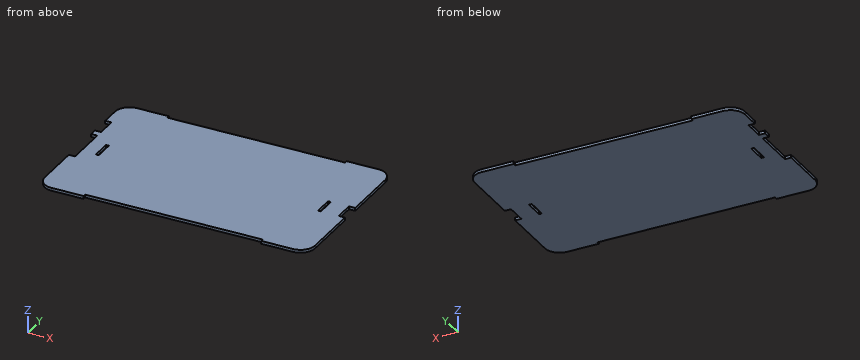
```python
from build123d import *

# Parameters (mm, degrees)
SALIENTE_EXTRUIR2_DEPTH = 3
CROQUIS2_W              = 6.5
CROQUIS2_H              = 20.5
CROQUIS2_H_2            = 44.2
CROQUIS2_W_2            = 3
CROQUIS2_H_3            = 20
CORTAR_EXTRUIR1_DEPTH   = 3


with BuildPart() as part:
    # Croquis1 → Saliente-Extruir2 (new body)
    with BuildSketch(Plane.XY):
        with BuildLine():
            Line((-207.344846765, 3), (-174.444846765, 3))
            Line((-174.444846765, 3), (-174.444846765, 0))
            Line((-174.444846765, 0), (9.755153235, 0))
            Line((9.755153235, 0), (9.755153235, 3))
            Line((9.755153235, 3), (42.655153235, 3))
            ThreePointArc((42.655153235, 3), (53.261754953, -1.393398282), (57.655153235, -12))
            Line((57.655153235, -12), (57.655153235, -152))
            ThreePointArc((57.655153235, -152), (53.261754953, -162.606601718), (42.655153235, -167))
            Line((42.655153235, -167), (9.755153235, -167))
            Line((9.755153235, -167), (9.755153235, -164))
            Line((9.755153235, -164), (-174.444846765, -164))
            Line((-174.444846765, -164), (-174.444846765, -167))
            Line((-174.444846765, -167), (-207.344846765, -167))
            ThreePointArc((-207.344846765, -167), (-217.951448483, -162.606601718), (-222.344846765, -152))
            Line((-222.344846765, -152), (-222.344846765, -12))
            ThreePointArc((-222.344846765, -12), (-217.951448483, -1.393398282), (-207.344846765, 3))
        make_face()
    extrude(amount=SALIENTE_EXTRUIR2_DEPTH)

    # Croquis2 → Cortar-Extruir1 (cut)
    with BuildSketch(Plane.XY.offset(3)):
        with Locations((-219.094846765, -42)):
            Rectangle(CROQUIS2_W, CROQUIS2_H)
        with Locations((-219.094846765, -82)):
            Rectangle(CROQUIS2_W, CROQUIS2_H_2)
        with Locations((54.405153235, -82)):
            Rectangle(CROQUIS2_W, CROQUIS2_H)
        with Locations((-199.094846765, -82)):
            Rectangle(CROQUIS2_W_2, CROQUIS2_H_3)
        with Locations((31.155153235, -82)):
            Rectangle(CROQUIS2_W_2, CROQUIS2_H_3)
    extrude(amount=-CORTAR_EXTRUIR1_DEPTH, mode=Mode.SUBTRACT)


solid = part.part
```
Part model, mm, in its own coordinate system. Round coordinates to 2 decimals unless told otherwise and drop trailing zeros. Write each loop counter-clockwise with the first axis right and the second up, starting at its lowest first coordinate (ties: lowest second). Pieces come first, ordered by that corner, then holes. Notation, with made-up numbers: (-12.75, 80) -> (19.25, 80) arc R21 ccw to (19.25, 108) -> close; hole circle Ø1 at (34, 40.5). An arc over 180 degrees is marked (long way). Return JSON: item names as keys, results as strings. Group by question number.
Q1. Pin check, flat tips, straight feed: pin 1 (1 mm diameter, centred on y = -34, z = 1, fed in from -X); pin 2 (12 mm diameter, centred on x = -136.5, y = -96.5, fed in from -Z); pin 3 (1 mm diameter, centred on x = -145, z = 1.5, fed in from -Y); pin 4 (1.5 mm diameter, centred on y = -165, z = 1.5, fed in from -X). Stop position of each tip, or through.
Q2. Saw through at B-B on x = -66. Write the cut outline in (y, z), plus the area to 3 significant figures.
Q3. Saw through at A-A on y = -83. Write the cut outline in (x, z).
Q4. Probe L1, parallel to X at y = -75, z = 0.3; L2, parallel to Y at x = -102, z = 0.9; L3, parallel to X at y = -40, z = 2. List the from-to ranges inside material, lowest first. Write a range as [from, to].
Q5. Saw through at C-C on z = 0.85. State how many separate pieces and enclosed holes the cut face has, plus the area to 3 significant figures.
Answer:
{
 "1": {"pin 1": "x = -215.84", "pin 2": "z = 0", "pin 3": "y = -164", "pin 4": "x = -216"},
 "2": {"outline": "(-164, 0) -> (0, 0) -> (0, 3) -> (-164, 3) -> close", "area": "492 mm2"},
 "3": {"outline": "(-215.84, 0) -> (-200.59, 0) -> (-200.59, 3) -> (-215.84, 3) -> close; (-197.59, 0) -> (29.66, 0) -> (29.66, 3) -> (-197.59, 3) -> close; (32.66, 0) -> (51.16, 0) -> (51.16, 3) -> (32.66, 3) -> close"},
 "4": {"L1": "[-215.84, -200.59], [-197.59, 29.66], [32.66, 51.16]", "L2": "[-164, 0]", "L3": "[-215.84, 57.66]"},
 "5": {"separate pieces": "1", "enclosed holes": "2", "area": "45,600 mm2"}
}
